```python
from build123d import *

# Parameters (mm, degrees)
SKETCH1_R           = 4.2
SKETCH1_R_2         = 2.05
BOSS_EXTRUDE1_DEPTH = 15


with BuildPart() as part:
    # Sketch1 → Boss-Extrude1 (new body)
    with BuildSketch(Plane.XY):
        with BuildLine():
            Line((-1.732050808, 52), (-4.758219757, 46.758521627))
            ThreePointArc((-4.758219757, 46.758521627), (-4.912837774, 46.742529082), (-5.067402052, 46.726025258))
            Line((-5.067402052, 46.726025258), (-9.117206581, 51.22378885))
            ThreePointArc((-9.117206581, 51.22378885), (-11.019319613, 51.841822839), (-12.505609264, 50.503561626))
            Line((-12.505609264, 50.503561626), (-14.375884531, 44.747446228))
            ThreePointArc((-14.375884531, 44.747446228), (-14.523798736, 44.699656266), (-14.671554076, 44.651377369))
            Line((-14.671554076, 44.651377369), (-19.567998292, 48.208852329))
            ThreePointArc((-19.567998292, 48.208852329), (-21.557042083, 48.417909255), (-22.732612588, 46.799875266))
            Line((-22.732612588, 46.799875266), (-23.365254167, 40.780692707))
            ThreePointArc((-23.365254167, 40.780692707), (-23.5, 40.703193978), (-23.634488785, 40.625250029))
            Line((-23.634488785, 40.625250029), (-29.163574581, 43.086957628))
            ThreePointArc((-29.163574581, 43.086957628), (-31.152618372, 42.877900702), (-31.966091658, 41.050809787))
            Line((-31.966091658, 41.050809787), (-31.333450078, 35.031627228))
            ThreePointArc((-31.333450078, 35.031627228), (-31.449138499, 34.927806797), (-31.564482923, 34.82360432))
            Line((-31.564482923, 34.82360432), (-37.484562718, 36.081956126))
            ThreePointArc((-37.484562718, 36.081956126), (-39.38667575, 35.463922137), (-39.802499132, 33.507626936))
            Line((-39.802499132, 33.507626936), (-37.932223865, 27.751511538))
            ThreePointArc((-37.932223865, 27.751511538), (-38.023798736, 27.625906858), (-38.114957694, 27.5))
            Line((-38.114957694, 27.5), (-44.167295593, 27.5))
            ThreePointArc((-44.167295593, 27.5), (-45.899346401, 26.5), (-45.899346401, 24.5))
            Line((-45.899346401, 24.5), (-42.873177451, 19.258521627))
            ThreePointArc((-42.873177451, 19.258521627), (-42.936636509, 19.116622225), (-42.999625918, 18.974513721))
            Line((-42.999625918, 18.974513721), (-48.919705713, 17.716161915))
            ThreePointArc((-48.919705713, 17.716161915), (-50.405995364, 16.377900702), (-49.990171982, 14.4216055))
            Line((-49.990171982, 14.4216055), (-45.940367454, 9.923841909))
            ThreePointArc((-45.940367454, 9.923841909), (-45.972937234, 9.771849468), (-46.005004154, 9.619750142))
            Line((-46.005004154, 9.619750142), (-51.53408995, 7.158042542))
            ThreePointArc((-51.53408995, 7.158042542), (-52.709660455, 5.540008553), (-51.896187168, 3.712917638))
            Line((-51.896187168, 3.712917638), (-46.999742952, 0.155442679))
            ThreePointArc((-46.999742952, 0.155442679), (-47, 0), (-46.999742952, -0.155442679))
            Line((-46.999742952, -0.155442679), (-51.896187168, -3.712917638))
            ThreePointArc((-51.896187168, -3.712917638), (-52.709660455, -5.540008553), (-51.53408995, -7.158042542))
            Line((-51.53408995, -7.158042542), (-46.005004154, -9.619750142))
            ThreePointArc((-46.005004154, -9.619750142), (-45.972937234, -9.771849468), (-45.940367454, -9.923841909))
            Line((-45.940367454, -9.923841909), (-49.990171982, -14.4216055))
            ThreePointArc((-49.990171982, -14.4216055), (-50.405995364, -16.377900702), (-48.919705713, -17.716161915))
            Line((-48.919705713, -17.716161915), (-42.999625918, -18.974513721))
            ThreePointArc((-42.999625918, -18.974513721), (-42.936636509, -19.116622225), (-42.873177451, -19.258521627))
            Line((-42.873177451, -19.258521627), (-45.899346401, -24.5))
            ThreePointArc((-45.899346401, -24.5), (-45.899346401, -26.5), (-44.167295593, -27.5))
            Line((-44.167295593, -27.5), (-38.114957694, -27.5))
            ThreePointArc((-38.114957694, -27.5), (-38.023798736, -27.625906858), (-37.932223865, -27.751511538))
            Line((-37.932223865, -27.751511538), (-39.802499132, -33.507626936))
            ThreePointArc((-39.802499132, -33.507626936), (-39.38667575, -35.463922137), (-37.484562718, -36.081956126))
            Line((-37.484562718, -36.081956126), (-31.564482923, -34.82360432))
            ThreePointArc((-31.564482923, -34.82360432), (-31.449138499, -34.927806797), (-31.333450078, -35.031627228))
            Line((-31.333450078, -35.031627228), (-31.966091658, -41.050809787))
            ThreePointArc((-31.966091658, -41.050809787), (-31.152618372, -42.877900702), (-29.163574581, -43.086957628))
            Line((-29.163574581, -43.086957628), (-23.634488785, -40.625250029))
            ThreePointArc((-23.634488785, -40.625250029), (-23.5, -40.703193978), (-23.365254167, -40.780692707))
            Line((-23.365254167, -40.780692707), (-22.732612588, -46.799875266))
            ThreePointArc((-22.732612588, -46.799875266), (-21.557042083, -48.417909255), (-19.567998292, -48.208852329))
            Line((-19.567998292, -48.208852329), (-14.671554076, -44.651377369))
            ThreePointArc((-14.671554076, -44.651377369), (-14.523798736, -44.699656266), (-14.375884531, -44.747446228))
            Line((-14.375884531, -44.747446228), (-12.505609264, -50.503561626))
            ThreePointArc((-12.505609264, -50.503561626), (-11.019319613, -51.841822839), (-9.117206581, -51.22378885))
            Line((-9.117206581, -51.22378885), (-5.067402052, -46.726025258))
            ThreePointArc((-5.067402052, -46.726025258), (-4.912837774, -46.742529082), (-4.758219757, -46.758521627))
            Line((-4.758219757, -46.758521627), (-1.732050808, -52))
            ThreePointArc((-1.732050808, -52), (0, -53), (1.732050808, -52))
            Line((1.732050808, -52), (4.758219757, -46.758521627))
            ThreePointArc((4.758219757, -46.758521627), (4.912837774, -46.742529082), (5.067402052, -46.726025258))
            Line((5.067402052, -46.726025258), (9.117206581, -51.22378885))
            ThreePointArc((9.117206581, -51.22378885), (11.019319613, -51.841822839), (12.505609264, -50.503561626))
            Line((12.505609264, -50.503561626), (14.375884531, -44.747446228))
            ThreePointArc((14.375884531, -44.747446228), (14.523798736, -44.699656266), (14.671554076, -44.651377369))
            Line((14.671554076, -44.651377369), (19.567998292, -48.208852329))
            ThreePointArc((19.567998292, -48.208852329), (21.557042083, -48.417909255), (22.732612588, -46.799875266))
            Line((22.732612588, -46.799875266), (23.365254167, -40.780692707))
            ThreePointArc((23.365254167, -40.780692707), (23.5, -40.703193978), (23.634488785, -40.625250029))
            Line((23.634488785, -40.625250029), (29.163574581, -43.086957628))
            ThreePointArc((29.163574581, -43.086957628), (31.152618372, -42.877900702), (31.966091658, -41.050809787))
            Line((31.966091658, -41.050809787), (31.333450078, -35.031627228))
            ThreePointArc((31.333450078, -35.031627228), (31.449138499, -34.927806797), (31.564482923, -34.82360432))
            Line((31.564482923, -34.82360432), (37.484562718, -36.081956126))
            ThreePointArc((37.484562718, -36.081956126), (39.38667575, -35.463922137), (39.802499132, -33.507626936))
            Line((39.802499132, -33.507626936), (37.932223865, -27.751511538))
            ThreePointArc((37.932223865, -27.751511538), (38.023798736, -27.625906858), (38.114957694, -27.5))
            Line((38.114957694, -27.5), (44.167295593, -27.5))
            ThreePointArc((44.167295593, -27.5), (45.899346401, -26.5), (45.899346401, -24.5))
            Line((45.899346401, -24.5), (42.873177451, -19.258521627))
            ThreePointArc((42.873177451, -19.258521627), (42.936636509, -19.116622225), (42.999625918, -18.974513721))
            Line((42.999625918, -18.974513721), (48.919705713, -17.716161915))
            ThreePointArc((48.919705713, -17.716161915), (50.405995364, -16.377900702), (49.990171982, -14.4216055))
            Line((49.990171982, -14.4216055), (45.940367454, -9.923841909))
            ThreePointArc((45.940367454, -9.923841909), (45.972937234, -9.771849468), (46.005004154, -9.619750142))
            Line((46.005004154, -9.619750142), (51.53408995, -7.158042542))
            ThreePointArc((51.53408995, -7.158042542), (52.709660455, -5.540008553), (51.896187168, -3.712917638))
            Line((51.896187168, -3.712917638), (46.999742952, -0.155442679))
            ThreePointArc((46.999742952, -0.155442679), (47, 0), (46.999742952, 0.155442679))
            Line((46.999742952, 0.155442679), (51.896187168, 3.712917638))
            ThreePointArc((51.896187168, 3.712917638), (52.709660455, 5.540008553), (51.53408995, 7.158042542))
            Line((51.53408995, 7.158042542), (46.005004154, 9.619750142))
            ThreePointArc((46.005004154, 9.619750142), (45.972937234, 9.771849468), (45.940367454, 9.923841909))
            Line((45.940367454, 9.923841909), (49.990171982, 14.4216055))
            ThreePointArc((49.990171982, 14.4216055), (50.405995364, 16.377900702), (48.919705713, 17.716161915))
            Line((48.919705713, 17.716161915), (42.999625918, 18.974513721))
            ThreePointArc((42.999625918, 18.974513721), (42.936636509, 19.116622225), (42.873177451, 19.258521627))
            Line((42.873177451, 19.258521627), (45.899346401, 24.5))
            ThreePointArc((45.899346401, 24.5), (45.899346401, 26.5), (44.167295593, 27.5))
            Line((44.167295593, 27.5), (38.114957694, 27.5))
            ThreePointArc((38.114957694, 27.5), (38.023798736, 27.625906858), (37.932223865, 27.751511538))
            Line((37.932223865, 27.751511538), (39.802499132, 33.507626936))
            ThreePointArc((39.802499132, 33.507626936), (39.38667575, 35.463922137), (37.484562718, 36.081956126))
            Line((37.484562718, 36.081956126), (31.564482923, 34.82360432))
            ThreePointArc((31.564482923, 34.82360432), (31.449138499, 34.927806797), (31.333450078, 35.031627228))
            Line((31.333450078, 35.031627228), (31.966091658, 41.050809787))
            ThreePointArc((31.966091658, 41.050809787), (31.152618372, 42.877900702), (29.163574581, 43.086957628))
            Line((29.163574581, 43.086957628), (23.634488785, 40.625250029))
            ThreePointArc((23.634488785, 40.625250029), (23.5, 40.703193978), (23.365254167, 40.780692707))
            Line((23.365254167, 40.780692707), (22.732612588, 46.799875266))
            ThreePointArc((22.732612588, 46.799875266), (21.557042083, 48.417909255), (19.567998292, 48.208852329))
            Line((19.567998292, 48.208852329), (14.671554076, 44.651377369))
            ThreePointArc((14.671554076, 44.651377369), (14.523798736, 44.699656266), (14.375884531, 44.747446228))
            Line((14.375884531, 44.747446228), (12.505609264, 50.503561626))
            ThreePointArc((12.505609264, 50.503561626), (11.019319613, 51.841822839), (9.117206581, 51.22378885))
            Line((9.117206581, 51.22378885), (5.067402052, 46.726025258))
            ThreePointArc((5.067402052, 46.726025258), (4.912837774, 46.742529082), (4.758219757, 46.758521627))
            Line((4.758219757, 46.758521627), (1.732050808, 52))
            ThreePointArc((1.732050808, 52), (0, 53), (-1.732050808, 52))
        make_face()
        Circle(SKETCH1_R, mode=Mode.SUBTRACT)
        with Locations((0, 8)):
            Circle(SKETCH1_R_2, mode=Mode.SUBTRACT)
        with Locations((8, 0)):
            Circle(SKETCH1_R_2, mode=Mode.SUBTRACT)
        with Locations((0, -8)):
            Circle(SKETCH1_R_2, mode=Mode.SUBTRACT)
        with Locations((-8, 0)):
            Circle(SKETCH1_R_2, mode=Mode.SUBTRACT)
    extrude(amount=BOSS_EXTRUDE1_DEPTH)


solid = part.part
```
The listing builds one solid part. Answer for the finished solid, in the listing's coordinates (mm). A direction names the side the tool comes from. Give positions to 0.01 mm unless a question says otherwise; leave off trailing zeros. Write each loop counter-clockwise with the first axis right and the second up, starting at its lowest first coordinate (ties: lowest second). Pieces come first, ordered by that corner, then holes. Notation, with made-up numbers: (1.5, -10) -> (36.5, -10) arc R27 ccw to (36.5, 12) -> close; hole circle Ø9 at (22.5, -23). An arc over 180 degrees is marked (long way). Use one line per item in the form item = value.
1) Each of these flat-tipped pins is pushed along its axis until it touches: P1, Ø6, axis at y = 20, z = 10, coming from the +X side; P2, Ø1, axis at y = -0.5, z = 9, coming from the +X side; P3, Ø4, axis at x = -22, z = 13, coming from the -Y side. Where does it stop, or does it pass through?
Result:
P1 = 50.07
P2 = 48.16
P3 = -48.59
2) Section B-B on z = 12 is taken. Count the separate pieces of the cut face and the enclosed holes in it, plus the area to 3 significant figures.
Result:
separate_pieces = 1
enclosed_holes = 5
area = 7,880 mm²
3) Section A-A on x = 0 is taken. Write down the section's boundary in (y, z).
Result:
outline = (-53, 0) -> (-10.05, 0) -> (-10.05, 15) -> (-53, 15) -> close; (-5.95, 0) -> (-4.2, 0) -> (-4.2, 15) -> (-5.95, 15) -> close; (4.2, 0) -> (5.95, 0) -> (5.95, 15) -> (4.2, 15) -> close; (10.05, 0) -> (53, 0) -> (53, 15) -> (10.05, 15) -> close
4) Straight lines are drawn through the part: probe 1 along X at (y, z) = (-48, 12); probe 2 along Y at (x, z) = (8, 4.25); probe 3 along Y at (x, z) = (48, 8.5). For each, find the intervals that lie inside material, in ascending order.
Result:
probe_1 = -22.16 to -19.28, -13.32 to -6.21, -4.04 to 4.04, 6.21 to 13.32, 19.28 to 22.16
probe_2 = -49.98 to -2.05, 2.05 to 49.98
probe_3 = -17.91 to -12.21, -8.73 to -0.88, 0.88 to 8.73, 12.21 to 17.91
5) A tool of negligible diameter and unlimited length cuts with its end or side. For faces 1 (the flat face through (23.053, 43.748, 7.395)), 2 (the flat face through (-23.053, -43.748, 7.395)), 3 (the flat face through (41, -27.5, 7)), 4 (the flat face through (-48.81, -8.37, 7.4)), from which of +Z, -Z, +X, -X, +Y, -Y can it reach the whole face along a straight path? Write none if from no direction.
Result:
face_1 = +Z, -Z, +Y
face_2 = +Z, -Z, -Y
face_3 = +Z, -Z, +X
face_4 = +Z, -Z, -X
6) Section D-D on y = -31 is taken. Write down the section's boundary in (x, z), plus the area to 3 significant figures.
Result:
outline = (-38.99, 0) -> (38.99, 0) -> (38.99, 15) -> (-38.99, 15) -> close
area = 1,170 mm²
7) Section C-C on x = 16 is taken. Write down the section's boundary in (y, z), plus the area to 3 significant figures.
Result:
outline = (-45.62, 0) -> (45.62, 0) -> (45.62, 15) -> (-45.62, 15) -> close
area = 1,370 mm²
8) For a pull along Y with two mould halves and no side action, classify faces 5 (the flat face through (-17.154, -46.455, 7.395)), 6 (the cylindrical face through (-45.9, -26.5, 7.4)), 7 (the cylindrical face through (5.95, 0.09, 7.4)), 8 (the flat face through (7.121, 49.006, 7.395)) as +Y half, -Y half, draft (parallel to the pull), parting line (faces both ways), or undercut.
Result:
face_5 = -Y half
face_6 = undercut
face_7 = undercut
face_8 = +Y half
